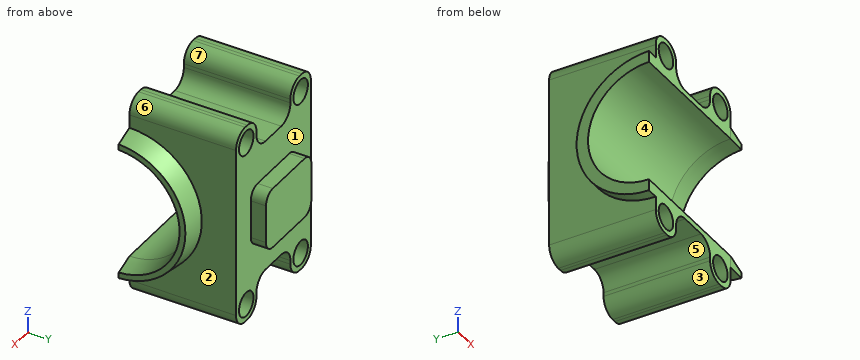
```python
from build123d import *

# Parameters (mm, degrees)
BOSS_EXTRUDE1_DEPTH  = 14
CUT_EXTRUDE1_REACH   = 22.967
SKETCH2_R            = 1.6
FILLET2_R            = 2
FILLET2_OF_MIRROR1_R = 2
BOSS_EXTRUDE2_DEPTH  = 2
CUT_EXTRUDE2_REACH   = 28.529
BOSS_EXTRUDE3_DEPTH  = 3
BOSS_EXTRUDE3_DRAFT  = 7
BOSS_EXTRUDE4_DEPTH  = 1.5


with BuildPart() as part:
    # Sketch1 → Boss-Extrude1 (new body)
    with BuildSketch(Plane(origin=(0, 0, 0), x_dir=(1, 0, 0), z_dir=(0, 1, 0))):
        Polygon((-8.25, 0), (-8.25, 13.25), (-3.75, 13.25), (-3.75, 8.75), (3.75, 8.75), (3.75, 13.25), (8.25, 13.25), (8.25, 0), align=None)
    boss_extrude1 = extrude(amount=BOSS_EXTRUDE1_DEPTH)

    # Sketch2 → Cut-Extrude1 (cut, up to next)
    with BuildSketch(Plane(origin=(0, 14, 0), x_dir=(1, 0, 0), z_dir=(0, 1, 0)), mode=Mode.PRIVATE) as cut_extrude1_sk1:
        with Locations(Location((-6, 11, 0), (0, 0, 270))):
            Circle(SKETCH2_R)
    cut_extrude1_tool1 = extrude(cut_extrude1_sk1.sketch, amount=-CUT_EXTRUDE1_REACH, mode=Mode.PRIVATE) & part.part
    # Sketch2 → Cut-Extrude1 (cut, up to next)
    with BuildSketch(Plane(origin=(0, 14, 0), x_dir=(1, 0, 0), z_dir=(0, 1, 0)), mode=Mode.PRIVATE) as cut_extrude1_sk2:
        with Locations(Location((6, 11, 0), (0, 0, 270))):
            Circle(SKETCH2_R)
    cut_extrude1_tool2 = extrude(cut_extrude1_sk2.sketch, amount=-CUT_EXTRUDE1_REACH, mode=Mode.PRIVATE) & part.part
    cut_extrude1_1 = cut_extrude1_tool1.solids().sort_by_distance((-6, 14, -11))[0]
    add(cut_extrude1_1, mode=Mode.SUBTRACT)
    cut_extrude1_2 = cut_extrude1_tool2.solids().sort_by_distance((6, 14, -11))[0]
    add(cut_extrude1_2, mode=Mode.SUBTRACT)
    cut_extrude1 = cut_extrude1_1 + cut_extrude1_2  # Cut-Extrude1 as one shape, for the pattern or mirror that repeats it

    # Fillet2
    fillet2_edges = [part.edges().sort_by_distance(p)[0] for p in [
        (-8.25, 7, -13.25),
        (-3.75, 7, -13.25),
        (-3.75, 7, -8.75),
        (3.75, 7, -8.75),
        (3.75, 7, -13.25),
        (8.25, 7, -13.25),
    ]]
    fillet(fillet2_edges, radius=FILLET2_R)

    # Mirror1: Boss-Extrude1, Cut-Extrude1 across plane
    add(boss_extrude1.mirror(Plane.XY))
    add(cut_extrude1.mirror(Plane.XY), mode=Mode.SUBTRACT)

    # Fillet2 of Mirror1
    fillet2_of_mirror1_edges = [part.edges().sort_by_distance(p)[0] for p in [
        (-8.25, 7, 13.25),
        (-3.75, 7, 13.25),
        (-3.75, 7, 8.75),
        (3.75, 7, 8.75),
        (3.75, 7, 13.25),
        (8.25, 7, 13.25),
    ]]
    fillet(fillet2_of_mirror1_edges, radius=FILLET2_OF_MIRROR1_R)

    # Sketch3 → Boss-Extrude2 (add)
    with BuildSketch(Plane(origin=(0, 14, 0), x_dir=(1, 0, 0), z_dir=(0, 1, 0))):
        with BuildLine():
            Line((-3.5, -4), (3.5, -4))
            ThreePointArc((3.5, -4), (4.560660172, -3.560660172), (5, -2.5))
            Line((5, -2.5), (5, 2.5))
            ThreePointArc((5, 2.5), (4.560660172, 3.560660172), (3.5, 4))
            Line((3.5, 4), (-3.5, 4))
            ThreePointArc((-3.5, 4), (-4.560660172, 3.560660172), (-5, 2.5))
            Line((-5, 2.5), (-5, -2.5))
            ThreePointArc((-5, -2.5), (-4.560660172, -3.560660172), (-3.5, -4))
        make_face()
    extrude(amount=BOSS_EXTRUDE2_DEPTH)

    # Sketch4 → Cut-Extrude2 (cut, up to next)
    with BuildSketch(Plane(origin=(8.25, 0, 0), x_dir=(0, 0, -1), z_dir=(1, 0, 0)), mode=Mode.PRIVATE) as cut_extrude2_sk1:
        with BuildLine():
            Line((-8, 0), (8, 0))
            ThreePointArc((8, 0), (0, 8), (-8, 0))
        make_face()
    cut_extrude2_tool1 = extrude(cut_extrude2_sk1.sketch, amount=-CUT_EXTRUDE2_REACH, mode=Mode.PRIVATE) & part.part
    add(cut_extrude2_tool1.solids().sort_by_distance((8.25, 3.395305, 0))[0], mode=Mode.SUBTRACT)


with BuildPart() as boss_extrude3_tool:
    # Sketch5 → Boss-Extrude3 (with draft: the straight prism first)
    with BuildSketch(Plane(origin=(8.25, 0, 0), x_dir=(0, 0, -1), z_dir=(1, 0, 0))):
        with BuildLine():
            Line((-9.5, 0), (-8, 0))
            ThreePointArc((-8, 0), (0, 8), (8, 0))
            Line((8, 0), (9.5, 0))
            ThreePointArc((9.5, 0), (0, 9.5), (-9.5, 0))
        make_face()
    extrude(amount=BOSS_EXTRUDE3_DEPTH)
    # Boss-Extrude3: the draft: its side faces are tilted about the plane it starts from
    boss_extrude3_sides = [boss_extrude3_tool.faces().sort_by_distance(p)[0] for p in [
        (9.75, 0, 8.75),
        (9.75, 8, 0),
        (9.75, 0, -8.75),
        (9.75, 9.5, 0),
    ]]
    draft(boss_extrude3_sides, Plane(origin=(8.25, 0, 0), x_dir=(0, 0, -1), z_dir=(1, 0, 0)), BOSS_EXTRUDE3_DRAFT)


with BuildPart() as part_1:
    add(part.part)

    # Boss-Extrude3: add boss_extrude3_tool
    add(boss_extrude3_tool.part)

    # Sketch6 → Boss-Extrude4 (add)
    with BuildSketch(Plane.ZY.offset(8.25)):
        with BuildLine():
            Line((-9.5, 0), (-8, 0))
            ThreePointArc((-8, 0), (0, 8), (8, 0))
            Line((8, 0), (9.5, 0))
            ThreePointArc((9.5, 0), (0, 9.5), (-9.5, 0))
        make_face()
    extrude(amount=BOSS_EXTRUDE4_DEPTH)


solid = part_1.part
```
Here's how the part is built. I have some questions about the finished solid (model axes, mm). Face numbers are marked on the shaded views. A direction names the side the tool comes from. Give positions to 0.01 mm unless a question says otherwise; leave off trailing zeros. Loops run counter-clockwise (first coordinate to the right, second up) from the corner with the lowest first, then second, coordinate; pieces in that order, holes last. Notation, with made-up numbers: (-11, 3) -> (9, 3) arc R24 ccw to (9, 22) -> close; hole circle Ø5 at (-18.5, -29). An arc over 180 degrees is marked (long way). Use one line per item in the form item = value. Start each with the question number.
1) Which directions (+Z, -Z, +X, -X, +Y, -Y) give clear straight access to the entire face, cutting with the end or side of a thin tool? Please do the marked faces 1, 2 and 3.
2) For P1, Ø3, axis at x = 6, z = -11, coming from the +Y side (3 decimals); P2, Ø1.5, axis at x = -4, z = 1, coming from the -Y side; P3, Ø1.6, axis at x = 1.5, y = 15, coming from the +Z side; P4, Ø1.5, axis at x = 7, z = 2.5, coming from the +Y side, each with a flat end and sliding along its axis, tell me the tip position at first contact or that it passes through.
3) Thinking about a two-plate mould opening in X: for the marked faces 4, 5, 6 and 7, which applies, +X half, -X half, draft (parallel to the pull), parting line (faces both ways), or undercut?
4) Imagine slicing it at B-B (y = 12). Please give me the cut outline in (x, z), then the cut area to 3 significant figures.
5) Please list where these lines run through material, in increasing order: line 1 along X through (y, z) = (5.25, -11); line 2 along Y through (x, z) = (-4.25, 5) (3 decimals); line 3 along Y through (x, z) = (3, -0.25).
6) Imagine slicing it at D-D (y = 2.5). Count the separate pieces of the cut face and the enclosed holes in it, then the cut area to 3 significant figures.
7) Imagine slicing it at A-A (x = -0.25). Please give me the cut outline in (y, z), then the cut area to 3 significant figures.
8) Imagine slicing it at C-C (z = 0). Please give me the cut outline in (x, y), then the cut area to 3 significant figures.
Check values:
q1.face_1 = +Y
q1.face_2 = +X, +Y
q1.face_3 = -Z, +Y, -Y
q2.P1 = through
q2.P2 = 7.81
q2.P3 = 4
q2.P4 = 14
q3.face_4 = draft
q3.face_5 = undercut
q3.face_6 = +X half
q3.face_7 = undercut
q4.outline = (-8.25, -11.25) arc R2 ccw to (-6.25, -13.25) -> (-5.75, -13.25) arc R2 ccw to (-3.75, -11.25) -> (-3.75, -10.75) arc R2 cw to (-1.75, -8.75) -> (1.75, -8.75) arc R2 cw to (3.75, -10.75) -> (3.75, -11.25) arc R2 ccw to (5.75, -13.25) -> (6.25, -13.25) arc R2 ccw to (8.25, -11.25) -> (8.25, 11.25) arc R2 ccw to (6.25, 13.25) -> (5.75, 13.25) arc R2 ccw to (3.75, 11.25) -> (3.75, 10.75) arc R2 cw to (1.75, 8.75) -> (-1.75, 8.75) arc R2 cw to (-3.75, 10.75) -> (-3.75, 11.25) arc R2 ccw to (-5.75, 13.25) -> (-6.25, 13.25) arc R2 ccw to (-8.25, 11.25) -> close; hole circle Ø3.2 at (-6, -11); hole circle Ø3.2 at (-6, 11); hole circle Ø3.2 at (6, -11); hole circle Ø3.2 at (6, 11)
q4.area = 334 mm^2
q5.line_1 = -8.25 to -7.6, -4.4 to -3.75, 3.75 to 4.4, 7.6 to 8.25
q5.line_2 = 6.245 to 14
q5.line_3 = 8 to 16
q6.separate_pieces = 2
q6.enclosed_holes = 4
q6.area = 95.2 mm^2
q7.outline = (0, -8.75) -> (14, -8.75) -> (14, -4) -> (16, -4) -> (16, 4) -> (14, 4) -> (14, 8.75) -> (0, 8.75) -> (0, 8) arc R8 cw to (0, -8) -> close
q7.area = 160 mm^2
q8.outline = (-9.75, 8) -> (8.25, 8) -> (11.25, 8.37) -> (11.25, 9.13) -> (8.25, 9.5) -> (8.25, 14) -> (5, 14) -> (5, 16) -> (-5, 16) -> (-5, 14) -> (-8.25, 14) -> (-8.25, 9.5) -> (-9.75, 9.5) -> close
q8.area = 125 mm^2
